Read the model definition and answer for the solid it produces. Units are mm, in the model's axes. Face numbers are marked on the shaded views. A direction names the side the tool comes from. Give positions to 0.01 mm unless a question says otherwise; leave off trailing zeros. Order: outer loops, then holes, each group sorted by start corner. A loop starts at its lowest first (then second) coordinate and runs counter-clockwise, first axis right, second up. Notation, with made-up numbers: (7.25, 72.5) -> (61.25, 72.5) arc R8 cw to (61.25, 86.5) -> close; hole circle Ø8 at (23.25, -30.75). An arc over 180 degrees is marked (long way). Use one line per item in the form item = value.
```python
from build123d import *

# Parameters (mm, degrees)
F1_DEPTH = 508
F3_D     = 26.9875
F3_DEPTH = 25.4
F4_D     = 26.9875
F4_DEPTH = 25.4


with BuildPart() as f1:
    # F0 (on Front) → F1 (new body, symmetric)
    with BuildSketch(Plane.XZ):
        with BuildLine():
            Line((127, -457.2), (127, -431.8))
            Line((127, -431.8), (12.065, -431.8))
            ThreePointArc((12.065, -431.8), (10.268949, -431.056051), (9.525, -429.26))
            Line((9.525, -429.26), (9.525, 429.26))
            ThreePointArc((9.525, 429.26), (10.268949, 431.056051), (12.065, 431.8))
            Line((12.065, 431.8), (127, 431.8))
            Line((127, 431.8), (127, 457.2))
            Line((127, 457.2), (-127, 457.2))
            Line((-127, 457.2), (-127, 431.8))
            Line((-127, 431.8), (-12.065, 431.8))
            ThreePointArc((-12.065, 431.8), (-10.268949, 431.056051), (-9.525, 429.26))
            Line((-9.525, 429.26), (-9.525, -429.26))
            ThreePointArc((-9.525, -429.26), (-10.268949, -431.056051), (-12.065, -431.8))
            Line((-12.065, -431.8), (-127, -431.8))
            Line((-127, -431.8), (-127, -457.2))
            Line((-127, -457.2), (127, -457.2))
        make_face()
    extrude(amount=F1_DEPTH, both=True)

    # F3
    with Locations(Plane.YZ.offset(9.525)):
        with Locations((92.075, 381), (92.075, 304.8), (92.075, 228.6), (92.075, 152.4)):
            Hole(F3_D / 2, depth=F3_DEPTH)

    # F4
    with Locations(Plane.YZ.offset(9.525)):
        with Locations((-92.075, 381), (-92.075, 304.8), (-92.075, 228.6), (-92.075, 152.4)):
            Hole(F4_D / 2, depth=F4_DEPTH)


solid = f1.part
```
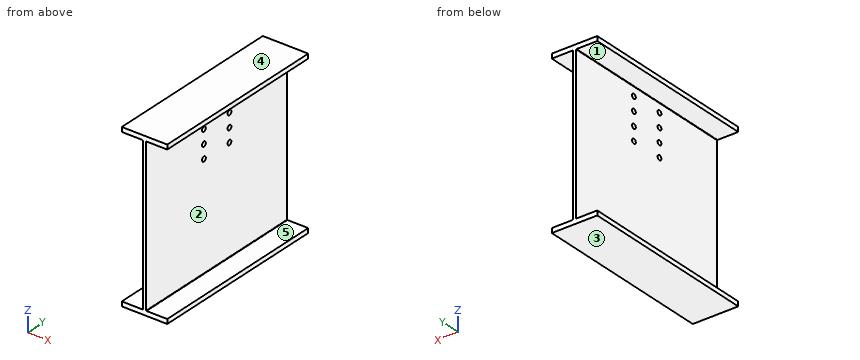
Item 1: The part is cut by section C-C on y = 338.5. Give the vertices of the cut face in (x, z) (3 decimals), and give its area (3 significant figures).
Checks:
outline = (-127, -457.2) -> (127, -457.2) -> (127, -431.8) -> (12.065, -431.8) arc R2.54 cw to (9.525, -429.26) -> (9.525, 429.26) arc R2.54 cw to (12.065, 431.8) -> (127, 431.8) -> (127, 457.2) -> (-127, 457.2) -> (-127, 431.8) -> (-12.065, 431.8) arc R2.54 cw to (-9.525, 429.26) -> (-9.525, -429.26) arc R2.54 cw to (-12.065, -431.8) -> (-127, -431.8) -> close
area = 29,400 mm²
Item 2: The part is cut by section B-B on x = 77. Give the vertices of the cut face in (y, z), and give its area (3 significant figures).
Checks:
outline = (-508, -457.2) -> (508, -457.2) -> (508, -431.8) -> (-508, -431.8) -> close; (-508, 431.8) -> (508, 431.8) -> (508, 457.2) -> (-508, 457.2) -> close
area = 51,600 mm²
Item 3: Determine the mould class of the marked faces 3, 4 and 5 for opening direction Z: +Z half, -Z half, draft (parallel to the pull), parting line (faces both ways), or undercut.
Checks:
face_3 = -Z half
face_4 = +Z half
face_5 = undercut
Item 4: Straight lines are drawn through the part: L1, parallel to Z at x = -108, y = -133; L2, parallel to X at y = -168, z = 228.5 (3 decimals); L3, parallel to Z at x = -10, y = -269.5. For each, find the intervals that lie inside material, in ascending order. Write a range as from..to.
Checks:
L1 = -457.2..-431.8, 431.8..457.2
L2 = -9.525..9.525
L3 = -457.2..-430.74, 430.74..457.2
Item 5: Given pin 1 Ø24.5 at (y, z) = (92.075, 304.8) entering from +X; pin 2 Ø1.5 at (y, z) = (94.5, 78.5) entering from -X (3 decimals); pin 3 Ø2 at (y, z) = (-396, 97.5) entering from +X (3 decimals), each flat-ended and moving along its own axis, determine where each tip first touches the part or whether it passes through.
Checks:
pin_1 = through
pin_2 = -9.525
pin_3 = 9.525
Item 6: The part is cut by section A-A on z = 381. Give the vertices of the cut face in (x, y) (3 decimals).
Checks:
outline = (-9.525, -508) -> (9.525, -508) -> (9.525, -105.569) -> (-9.525, -105.569) -> close; (-9.525, -78.581) -> (9.525, -78.581) -> (9.525, 78.581) -> (-9.525, 78.581) -> close; (-9.525, 105.569) -> (9.525, 105.569) -> (9.525, 508) -> (-9.525, 508) -> close
Item 7: The part is cut by section D-D on z = -79. Give the vertices of the cut face in (x, y) (3 decimals), and give its area (3 significant figures).
Checks:
outline = (-9.525, -508) -> (9.525, -508) -> (9.525, 508) -> (-9.525, 508) -> close
area = 19,400 mm²
Item 8: Which of the six approach directions +Z, -Z, +X, -X, +Y, -Y give full straight-line access (tool end or side, diameter ignored) to the marked faces 1 and 2?
Checks:
face_1 = -X, +Y, -Y
face_2 = +X, +Y, -Y
